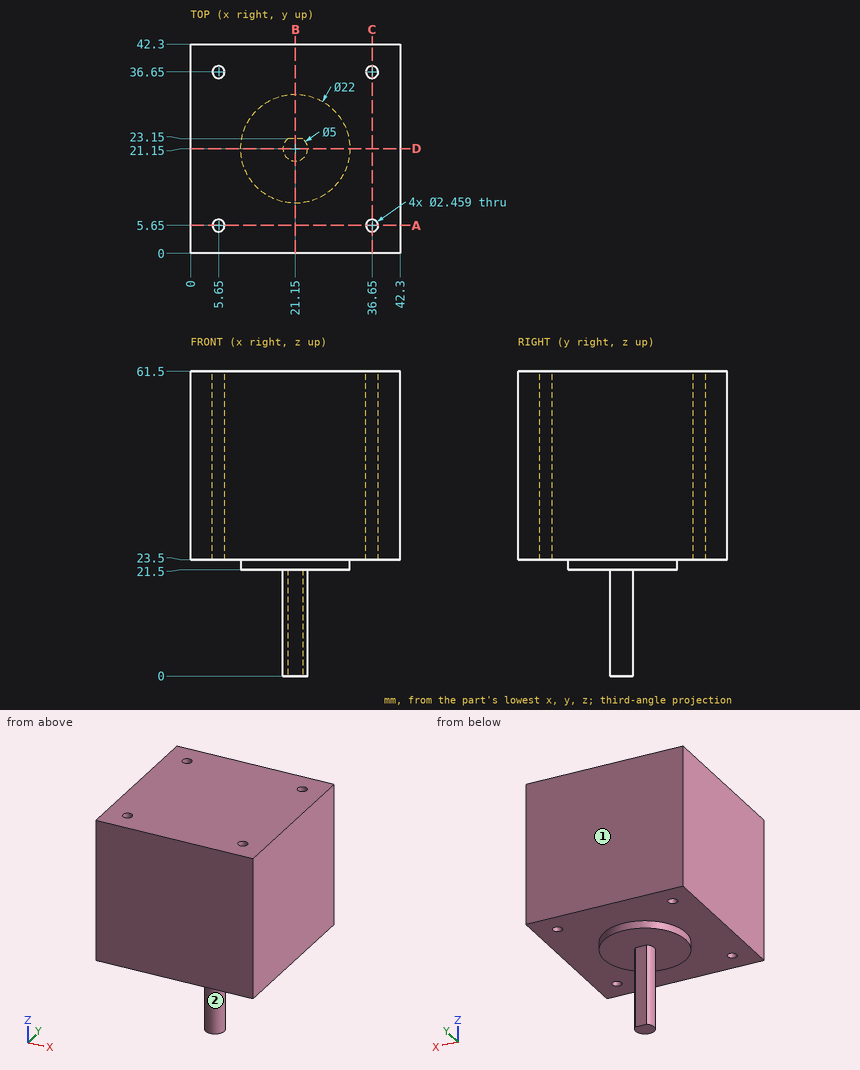
Study the drawing (mm; zero at the part's minimum x, y, z) and answer. A direction names the side the tool comes from. Give positions to 0.01 mm unless a question says otherwise; leave off trailing zeros. Write each loop counter-clockwise with the first axis right and the second up, starting at its lowest first coordinate (ties: lowest second). Pieces come first, ordered by that corner, then holes. Notation, with made-up numbers: (8, 52) - (59, 52) arc R13 ccw to (59, 71) - close; hole circle Ø9 at (-31.75, 41). An arc over 180 degrees is marked (long way). One line per question, with ' | ' between items. Start each with the question number.
1. Section B-B, the plane x = 21.15 is taken. Determine the outline of the cut face in (y, z).
2. Given P1, Ø1, axis at x = 6.5, y = 38, coming from the -Z side; P2, Ø0.9, axis at x = 21, z = 6.5, coming from the +Y side; P3, Ø1.5, axis at x = 22.5, y = 24, coming from the -Z side; P4, Ø1.5, axis at x = 5.65, y = 5.65, coming from the +Z side, each flat-ended and moving along its own axis, determine where each tip first touches the part or whether it passes through.
3. For the marked faces 1 and 2, determine the directions among +Z, -Z, +X, -X, +Y, -Y from which every point of the face is accessible in a straight line to the end or side of a thin tool.
4. Section D-D, the plane y = 21.15 is taken. Determine the outline of the cut face in (x, z).
5. Section A-A, the plane y = 5.65 is taken. Determine the outline of the cut face in (x, z), then the cut area to 3 significant figures.
6. Straight lines are drawn through the part: line 1 (Y direction, x = 5.65, z = 44); line 2 (X direction, y = 36, z = 32). For each, find the intervals that lie inside material, in ascending order.
Result:
1) outline: (0, 23.5) - (10.15, 23.5) - (10.15, 21.5) - (18.65, 21.5) - (18.65, 0) - (23.15, 0) - (23.15, 21.5) - (32.15, 21.5) - (32.15, 23.5) - (42.3, 23.5) - (42.3, 61.5) - (0, 61.5) - close
2) P1: stops at z = 23.5 | P2: stops at y = 23.15 | P3: stops at z = 21.5 | P4: passes through
3) face 1: +Z, -Z, +X, -X, +Y | face 2: -Z
4) outline: (0, 23.5) - (10.15, 23.5) - (10.15, 21.5) - (18.65, 21.5) - (18.65, 0) - (23.65, 0) - (23.65, 21.5) - (32.15, 21.5) - (32.15, 23.5) - (42.3, 23.5) - (42.3, 61.5) - (0, 61.5) - close
5) outline: (0, 23.5) - (4.42, 23.5) - (4.42, 61.5) - (0, 61.5) - close; (6.88, 23.5) - (35.42, 23.5) - (35.42, 61.5) - (6.88, 61.5) - close; (37.88, 23.5) - (42.3, 23.5) - (42.3, 61.5) - (37.88, 61.5) - close | area: 1,420 mm2
6) line 1: y = 0 to 4.42, 6.88 to 35.42, 37.88 to 42.3 | line 2: x = 0 to 4.61, 6.69 to 35.61, 37.69 to 42.3
